```python
from build123d import *

# Parameters (mm, degrees)
SKETCH1_W           = 55
SKETCH1_H           = 28
BOSS_EXTRUDE1_DEPTH = 1.5
SKETCH4_R           = 1.5
CUT_EXTRUDE1_DEPTH  = 38.262581768


with BuildPart() as part:
    # Sketch1 → Boss-Extrude1 (new body)
    with BuildSketch(Plane(origin=(0, 0, 0), x_dir=(1, 0, 0), z_dir=(0, 1, 0))):
        Rectangle(SKETCH1_W, SKETCH1_H)
        with BuildLine():
            Line((-27.5, -7), (-27.5, 7))
            ThreePointArc((-27.5, 7), (-34.5, 0), (-27.5, -7))
        make_face()
        with BuildLine():
            ThreePointArc((27.5, -7), (34.5, 0), (27.5, 7))
            Line((27.5, 7), (27.5, -7))
        make_face()
    extrude(amount=-BOSS_EXTRUDE1_DEPTH)

    # Sketch4 → Cut-Extrude1 (cut, through all)
    with BuildSketch(Plane(origin=(0, 0, 0), x_dir=(1, 0, 0), z_dir=(0, 1, 0))):
        with Locations(Location((-31.49, 0, 0), (0, 0, 270))):
            Circle(SKETCH4_R)
        with Locations(Location((31.49, 0, 0), (0, 0, 270))):
            Circle(SKETCH4_R)
    extrude(amount=-CUT_EXTRUDE1_DEPTH, mode=Mode.SUBTRACT)


solid = part.part
```
Geometry check sheet. Reference: the model listing, model coordinates, mm. A direction names the side the tool comes from. Give positions to 0.01 mm unless a question says otherwise; leave off trailing zeros. Write each loop counter-clockwise with the first axis right and the second up, starting at its lowest first coordinate (ties: lowest second). Pieces come first, ordered by that corner, then holes. Notation, with made-up numbers: (88, -38) -> (121, -38) arc R18 ccw to (121, -11) -> close; hole circle Ø8 at (15, -6.75). An arc over 180 degrees is marked (long way). One line per question, with ' | ' between items.
Item 1: Sectioned sample at C-C, the plane x = 31.49. Record the boundary of the cut face in (y, z), plus the area to 3 significant figures.
Determined:
outline: (-1.5, -5.75) -> (0, -5.75) -> (0, -1.5) -> (-1.5, -1.5) -> close; (-1.5, 1.5) -> (0, 1.5) -> (0, 5.75) -> (-1.5, 5.75) -> close | area: 12.8 mm^2
Item 2: Sectioned sample at D-D, the plane z = 8.5. Record the boundary of the cut face in (x, y).
Determined:
outline: (-27.5, -1.5) -> (27.5, -1.5) -> (27.5, 0) -> (-27.5, 0) -> close
Item 3: Sectioned sample at B-B, the plane z = 0. Record the boundary of the cut face in (x, y).
Determined:
outline: (-34.5, -1.5) -> (-32.99, -1.5) -> (-32.99, 0) -> (-34.5, 0) -> close; (-29.99, -1.5) -> (29.99, -1.5) -> (29.99, 0) -> (-29.99, 0) -> close; (32.99, -1.5) -> (34.5, -1.5) -> (34.5, 0) -> (32.99, 0) -> close
Item 4: Scan lines: line 1 along X through (y, z) = (-1, 0); line 2 along X through (y, z) = (-0.6, 1); line 3 along X through (y, z) = (-0.3, 8.5). Record each from-to range of solid material in increasing order.
Determined:
line 1: -34.5 to -32.99, -29.99 to 29.99, 32.99 to 34.5 | line 2: -34.43 to -32.61, -30.37 to 30.37, 32.61 to 34.43 | line 3: -27.5 to 27.5
Item 5: Access from +Z, -Z, +X, -X, +Y, -Y to the whole of each face (thin tool, end or side, straight path). Record for faces 1 (the flat face through (-27.5, -1, -10)), 2 (the flat face through (27.5, -1, 11)), 3 (the flat face through (-27.5, -1, 11)).
Determined:
face 1: -Z, -X, +Y, -Y | face 2: +Z, +X, +Y, -Y | face 3: +Z, -X, +Y, -Y
Item 6: Sectioned sample at A-A, the plane y = -1.1. Record the boundary of the cut face in (x, z).
Determined:
outline: (-27.5, -14) -> (27.5, -14) -> (27.5, -7) arc R7 ccw to (27.5, 7) -> (27.5, 14) -> (-27.5, 14) -> (-27.5, 7) arc R7 ccw to (-27.5, -7) -> close; hole circle Ø3 at (-31.49, 0); hole circle Ø3 at (31.49, 0)
Item 7: Draft check along X on faces 4 (the cylindrical face through (32.977, -0.74, -0.195)), 5 (the flat face through (0, 0, 0)), 6 (the flat face through (27.5, -1, -10)). Enter one of: released by +X, released by -X, zero draft, split by the parting line, or undercut.
Determined:
face 4: undercut | face 5: zero draft | face 6: released by +X
